Can you work these out from the model? Positions are in its coordinate system, mm. Give positions to 0.01 mm unless a question says otherwise; leave off trailing zeros. Write each question's results on one line, items separated by ' | '. Start each with the question number.
from build123d import *

# Parameters (mm, degrees)
SKETCH1_W                                        = 203.2
SKETCH1_H                                        = 152.4
BOSS_EXTRUDE1_DEPTH                              = 12.7
CSK_FOR_3_8_FLAT_HEAD_MACHINE_SCREW1_D           = 9.8044
CSK_FOR_3_8_FLAT_HEAD_MACHINE_SCREW1_CSINK_D     = 19.3548
CSK_FOR_3_8_FLAT_HEAD_MACHINE_SCREW1_CSINK_ANGLE = 82


with BuildPart() as part:
    # Sketch1 → Boss-Extrude1 (new body)
    with BuildSketch(Plane.XY):
        Rectangle(SKETCH1_W, SKETCH1_H)
    extrude(amount=BOSS_EXTRUDE1_DEPTH)

    # CSK for 3/8 Flat Head Machine Screw1 (through all)
    with Locations(Plane.XY.offset(12.7)):
        with Locations((-92.075, 57.15), (-92.075, -57.15), (92.075, -57.15), (92.075, 57.15), (-92.075, 19.05), (92.075, 19.05), (92.075, -19.05), (-92.075, -19.05)):
            CounterSinkHole(CSK_FOR_3_8_FLAT_HEAD_MACHINE_SCREW1_D / 2, CSK_FOR_3_8_FLAT_HEAD_MACHINE_SCREW1_CSINK_D / 2, counter_sink_angle=CSK_FOR_3_8_FLAT_HEAD_MACHINE_SCREW1_CSINK_ANGLE)


solid = part.part
Q1. If I drill on probe 1 along X at (y, z) = (57.15, 5); probe 2 along X at (y, z) = (-20.5, 4.25), over which ranges is the centre line in solid material (lowest first)? Write a range as from..to.
Q2. Will these pins go through, and if not, where does the flat tip stop? P1, Ø15.5, axis at x = -92.075, y = -19.05, coming from the +Z side; P2, Ø11.5, axis at x = -92.075, y = 57.15, coming from the +Z side.
Q3. Thinking about a two-plate mould opening in X: for faces 1 (the flat face through (-1, -76.2, 6)), 2 (the conical face through (97.2, -18.82, 7.47)), which applies, released by +X, released by -X, zero draft, split by the parting line, or undercut?
Q4. If we section it at A-A (z = 2): State how many separate pieces and enclosed holes the cut face has, plus the area to 3 significant figures.
Findings below:
1) probe 1: x = -101.6..-96.98, -87.17..87.17, 96.98..101.6 | probe 2: x = -101.6..-96.76, -87.39..87.39, 96.76..101.6
2) P1: stops at z = 10.48 | P2: stops at z = 8.18
3) face 1: zero draft | face 2: undercut
4) separate pieces: 1 | enclosed holes: 8 | area: 30,400 mm2
